Check sheet for the modelled part. Datum: model origin and axes. Units: mm. Coordinates: 2 decimals unless noted, no trailing zeros. Loops run counter-clockwise (first coordinate to the right, second up) from the corner with the lowest first, then second, coordinate; pieces in that order, holes last. Notation, with made-up numbers: (-6.5, 77.25) -> (11.5, 77.25) arc R19 cw to (11.5, 95.25) -> close; hole circle Ø10 at (-19, 86). An arc over 180 degrees is marked (long way). Use one line per item in the form item = value.
Autodesk Inventor part; units mm, degrees
ref_plane "YZ Plane" through (0, 0, 0) normal (1, 0, 0) x (0, 1, 0)
ref_plane "XZ Plane" through (0, 0, 0) normal (0, 1, 0) x (-1, 0, 0)
ref_plane "XY Plane" through (0, 0, 0) normal (0, 0, 1) x (1, 0, 0)
sketch "Sketch1" plane through (0, 0, 0) normal (0, 1, 0) x (-1, 0, 0)
  line L0 (-7, 17) -> (7, 17)
  line L1 (17, 7) -> (17, -7)
  line L2 (7, -17) -> (-7, -17)
  line L3 (-17, -7) -> (-17, 7)
  line L4 (-17, 17) -> (17, -17) construction
  line L5 (17, 17) -> (-17, -17) construction
  arc A0 (17, 7) -> (7, 17) centre (7, 7) ccw
  arc A1 (7, -17) -> (17, -7) centre (7, -7) ccw
  arc A2 (-17, -7) -> (-7, -17) centre (-7, -7) ccw
  arc A3 (-7, 17) -> (-17, 7) centre (-7, 7) ccw
  line L6 (-7, -22) -> (7, -22)
  arc A4 (7, -22) -> (22, -7) centre (7, -7) ccw
  line L7 (22, -7) -> (22, 7)
  arc A5 (22, 7) -> (7, 22) centre (7, 7) ccw
  line L8 (7, 22) -> (-7, 22)
  arc A6 (-7, 22) -> (-22, 7) centre (-7, 7) ccw
  line L9 (-22, 7) -> (-22, -7)
  arc A7 (-22, -7) -> (-7, -22) centre (-7, -7) ccw
  circle A8 centre (-15.8388, -15.8388) radius 1.05
  line L10 (-14.0711, -14.0711) -> (-17.6066, -17.6066) construction
  circle A9 centre (15.8388, -15.8388) radius 1.05
  circle A10 centre (15.8388, 15.8388) radius 1.05
  circle A11 centre (-15.8388, 15.8388) radius 1.05
  line L11 (14.5, -7) -> (14.5, 7)
  arc A12 (14.5, 7) -> (7, 14.5) centre (7, 7) ccw
  line L12 (7, 14.5) -> (-7, 14.5)
  arc A13 (-7, 14.5) -> (-14.5, 7) centre (-7, 7) ccw
  line L13 (-14.5, 7) -> (-14.5, -7)
  arc A14 (-14.5, -7) -> (-7, -14.5) centre (-7, -7) ccw
  line L14 (-7, -14.5) -> (7, -14.5)
  arc A15 (7, -14.5) -> (14.5, -7) centre (7, -7) ccw
  point P0 (0, 0)
  dimension "d0" = 34
  dimension "d1" = 34
  dimension "d2" = 10
  dimension "d3" = 5
  dimension "d4" = 2.1
  dimension "d7" = 360
  dimension "d11" = 2.5
extrude "Extrusion1" add sketch "Sketch1" along normal blind 2.75 contours A7 L9 A6 L8 A5 L7 A4 L6
extrude "Extrusion2" add sketch "Sketch1" against normal blind 2.5 contours L0 A0 L1 A1 L2 A2 L3 A3 | A7 L9 A6 L8 A5 L7 A4 L6
chamfer "Chamfer1" distance 1 distance2 2.5 8 edges at (17.6066, -2.5, 17.6066) (0, -2.5, 22) (-17.6066, -2.5, 17.6066) (-22, -2.5, 0) (-17.6066, -2.5, -17.6066) (0, -2.5, -22) (17.6066, -2.5, -17.6066) (22, -2.5, 0) measured on face at (19.5, -2.5, 2.3333)
properties part number "subcap"
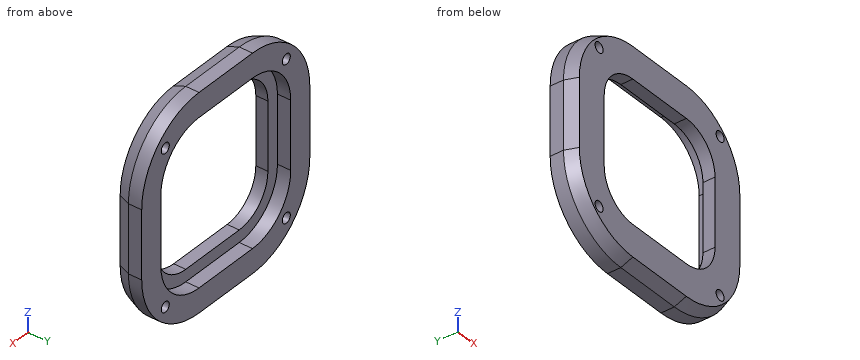
(1) Section check A-A, the plane x = -5.5. Record the boundary of the cut face in (y, z), plus the area to 3 significant figures.
Established:
outline = (-2.5, -21) -> (0, -22) -> (2.75, -22) -> (2.75, -17) -> (0, -17) -> (0, -14.5) -> (-2.5, -14.5) -> close; (-2.5, 14.5) -> (0, 14.5) -> (0, 17) -> (2.75, 17) -> (2.75, 22) -> (0, 22) -> (-2.5, 21) -> close
area = 62.5 mm²
(2) Scan lines: line 1 along X through (y, z) = (0.95, -2); line 2 along X through (y, z) = (-0.25, -16). Record each from-to range of solid material in increasing order.
Established:
line_1 = -22 to -17, 17 to 22
line_2 = -18.87 to -16.88, -14.8 to 14.8, 16.88 to 18.87
(3) Section check B-B, the plane z = 2.5. Record the boundary of the cut face in (x, y).
Established:
outline = (-22, 0) -> (-21, -2.5) -> (-14.5, -2.5) -> (-14.5, 0) -> (-17, 0) -> (-17, 2.75) -> (-22, 2.75) -> close; (14.5, -2.5) -> (21, -2.5) -> (22, 0) -> (22, 2.75) -> (17, 2.75) -> (17, 0) -> (14.5, 0) -> close
(4) Section check C-C, the plane y = 2.2. Record the boundary of the cut face in (x, z).
Established:
outline = (-22, -7) arc R15 ccw to (-7, -22) -> (7, -22) arc R15 ccw to (22, -7) -> (22, 7) arc R15 ccw to (7, 22) -> (-7, 22) arc R15 ccw to (-22, 7) -> close; hole (-17, -7) arc R10 ccw to (-7, -17) -> (7, -17) arc R10 ccw to (17, -7) -> (17, 7) arc R10 ccw to (7, 17) -> (-7, 17) arc R10 ccw to (-17, 7) -> close; hole circle Ø2.1 at (-15.84, -15.84); hole circle Ø2.1 at (-15.84, 15.84); hole circle Ø2.1 at (15.84, -15.84); hole circle Ø2.1 at (15.84, 15.84)
(5) Section check D-D, the plane y = -1.6. Record the boundary of the cut face in (x, z).
Established:
outline = (-21.36, -7) arc R14.36 ccw to (-7, -21.36) -> (7, -21.36) arc R14.36 ccw to (21.36, -7) -> (21.36, 7) arc R14.36 ccw to (7, 21.36) -> (-7, 21.36) arc R14.36 ccw to (-21.36, 7) -> close; hole circle Ø2.1 at (-15.84, -15.84); hole circle Ø2.1 at (-15.84, 15.84); hole (-14.5, -7) arc R7.5 ccw to (-7, -14.5) -> (7, -14.5) arc R7.5 ccw to (14.5, -7) -> (14.5, 7) arc R7.5 ccw to (7, 14.5) -> (-7, 14.5) arc R7.5 ccw to (-14.5, 7) -> close; hole circle Ø2.1 at (15.84, -15.84); hole circle Ø2.1 at (15.84, 15.84)
(6) Go/stop test with flat-tipped pins: P1, Ø2.5, axis at x = -15.84, z = -15.84, coming from the +Y side; P2, Ø1.2, axis at x = -0.5, y = -1.5, coming from the +Z side; P3, Ø3, axis at x = -10, y = 2, coming from the +Z side. Record where each tip stops, or that it passes through.
Established:
P1 = 2.75
P2 = 21.64
P3 = 21.92
